```python
from build123d import *

# Parameters (mm, degrees)
F0_W             = 140
F0_H             = 50
F1_DEPTH         = 8
F3_D             = 12
F4_D             = 5.5
F5_D             = 7
F6_D             = 18.5
F7_D             = 4.4
F7_COPIES_COUNT  = 4
F7_COPIES4_COUNT = 2
F7_COPIES4_PITCH = 62.25753


# Not quite as in the source:
# - a pattern or mirror of a feature is missing from the dataset's text; its kind, count and spacing are read off the source's solid


with BuildPart() as f1:
    # F0 (on Front) → F1 (new body)
    with BuildSketch(Plane.XZ):
        Rectangle(F0_W, F0_H)
    extrude(amount=F1_DEPTH)

    # F3 (through all)
    with Locations(Plane.XZ.offset(8)):
        with Locations((0, 0)):
            Hole(F3_D / 2)

    # F4 (through all)
    with Locations(Plane.XZ.offset(8)):
        with Locations((-7, 7), (-7, -7), (7, -7), (7, 7)):
            Hole(F4_D / 2)

    # F5 (through all)
    with Locations(Plane.XZ.offset(8)):
        with Locations((-62.5, -17.5), (62.5, -17.5), (62.5, 17.5), (-62.5, 17.5)):
            Hole(F5_D / 2)

    # F6 (through all)
    with Locations(Plane.XZ.offset(8)):
        with Locations((-29, 0), (29, 0)):
            Hole(F6_D / 2)

    # F7 (through all)
    with Locations(Plane.XZ.offset(8)):
        with Locations((-40.313708499, 11.313708499)):
            f7 = Hole(F7_D / 2)

    # F7_copies: F7 ×4 about axis
    f7_copies_axis = Axis((-29, 0, 0), (0, 1, 0))
    for i in range(1, F7_COPIES_COUNT):
        add(f7.rotate(f7_copies_axis, i * 360 / F7_COPIES_COUNT), mode=Mode.SUBTRACT)

    # F7_copies1: F7 across plane
    add(f7.mirror(Plane(origin=(0, 0, 0), x_dir=(0, 0, 1), z_dir=(1, 0, 0))), mode=Mode.SUBTRACT)

    # F7_copies2: F7 across plane
    add(f7.mirror(Plane(origin=(-11.313708, 0, 0), x_dir=(0, 0, 1), z_dir=(1, 0, 0))), mode=Mode.SUBTRACT)

    # F7_copies3: F7 across plane
    add(f7.mirror(Plane(origin=(0, 0, 0), x_dir=(0.2702028103, 0, 0.9628034282), z_dir=(0.9628034282, 0, -0.2702028103))), mode=Mode.SUBTRACT)

    # F7_copies4: F7 ×2
    with Locations(*[Vector(0.931614221, 0, -0.3634486803) * (i * F7_COPIES4_PITCH) for i in range(1, F7_COPIES4_COUNT)]):
        add(f7, mode=Mode.SUBTRACT)


solid = f1.part
```
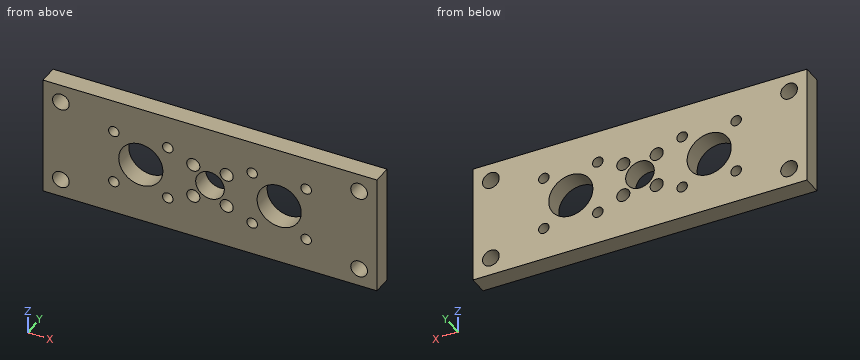
Read the model definition and answer for the solid it produces. Units are mm, in the model's axes. Round coordinates to 2 decimals unless told otherwise and drop trailing zeros. Loops run counter-clockwise (first coordinate to the right, second up) from the corner with the lowest first, then second, coordinate; pieces in that order, holes last. Notation, with made-up numbers: (35.5, 45) -> (45.5, 45) arc R9 ccw to (45.5, 60) -> close; hole circle Ø6 at (-27, 83). An arc over 180 degrees is marked (long way). One line per item, written item: value.
1) A cutting plane is placed at A-A (z = -17.5). Determine the outline of the cut face in (x, y), and give its area (3 significant figures).
Answer list:
outline: (-70, -8) -> (-66, -8) -> (-66, 0) -> (-70, 0) -> close; (-59, -8) -> (59, -8) -> (59, 0) -> (-59, 0) -> close; (66, -8) -> (70, -8) -> (70, 0) -> (66, 0) -> close
area: 1,010 mm²
2) A cutting plane is placed at B-B (x = 0). Determine the outline of the cut face in (y, z).
Answer list:
outline: (-8, -25) -> (0, -25) -> (0, -6) -> (-8, -6) -> close; (-8, 6) -> (0, 6) -> (0, 25) -> (-8, 25) -> close
3) A cutting plane is placed at D-D (y = -5.75). Give the number of separate pieces and of enclosed holes in the cut face, and give its area (3 significant figures).
Answer list:
separate pieces: 1
enclosed holes: 19
area: 5,980 mm²
4) Consider L1, parallel to Z at x = 62.5, y = -4.5; L2, parallel to X at y = -5.5, z = 4.5; L3, parallel to Z at x = 0, y = -1. Determine where each line is inside the solid, lowest interval first. Write a range as [from, to].
Answer list:
L1: z = [-25, -21], [-14, 14], [21, 25]
L2: x = [-70, -37.08], [-20.92, -8.15], [-5.85, -3.97], [3.97, 5.85], [8.15, 20.92], [37.08, 70]
L3: z = [-25, -6], [6, 25]
5) A cutting plane is placed at C-C (z = -2.5). Determine the outline of the cut face in (x, y), and give its area (3 significant figures).
Answer list:
outline: (-70, -8) -> (-37.91, -8) -> (-37.91, 0) -> (-70, 0) -> close; (-20.09, -8) -> (-5.45, -8) -> (-5.45, 0) -> (-20.09, 0) -> close; (5.45, -8) -> (20.09, -8) -> (20.09, 0) -> (5.45, 0) -> close; (37.91, -8) -> (70, -8) -> (70, 0) -> (37.91, 0) -> close
area: 748 mm²
